Can you work these out from the model? Positions are in its coordinate system, mm. A direction names the side the tool comes from. Coordinates: 2 decimals unless noted, no trailing zeros. Order: outer loops, then holes, each group sorted by start corner. A loop starts at its lowest first (then second) coordinate and runs counter-clockwise, first axis right, second up. Notation, with made-up numbers: (39.25, 14.25) - (83.25, 14.25) arc R17 ccw to (83.25, 39.25) - close; hole circle Ø8 at (14, 51). An arc over 180 degrees is marked (long way). Return JSON: item names as keys, results as strings. Group by question number.
1) Imagine slicing it at A-A (y = 27.02). Write out the boundary of the cut face in (x, z), and give its area (3 significant figures).
2) If I drill on line 1 along Z through (x, y) = (104, 42); line 2 along Y through (x, z) = (33.5, 172.5); line 3 along Z through (x, y) = (64, 43), over which ranges is the centre line in solid material (lowest first)?
3) If we mould it in two halves opening along X, with no side actions, what happens to faces 6 (the face through (9.191, 2.535, 258.964)), 7 (the face through (203.746, 2, 211)), 8 (the face through (154, 2, 266.465))? For each: pulls with the +X half, pulls with the -X half, needs draft (parallel to the pull), parting line crosses it, or undercut.
4) Imagine slicing it at C-C (x = 30). Write out the boundary of the cut face in (y, z), and give its area (3 significant figures).
5) For pin 1 Ø5.5 at (y, z) = (3.5, 272.5) entering from -X; pin 2 Ø1 at (y, z) = (11, 246.5) entering from -X; pin 3 Ø8 at (x, z) = (20, 251.5) entering from -Y; pin 4 Ø8 at (x, z) = (173.5, 82.5) entering from +Y, each with a flat end and sliding along its axis, tell me the tip position at first contact or that it passes through.
6) Which directions (+Z, -Z, +X, -X, +Y, -Y) give clear straight access to the entire face, cutting with the end or side of a thin tool? Please do faces 1 (the face through (17.947, 2.535, 261.535)), 2 (the face through (16, 2.5, 81)), 3 (the face through (88, 49.05, 252)), 4 (the face through (172, 2.5, 81)), 5 (the face through (206, 2, 226.465)).
7) Imagine slicing it at D-D (z = 115). Write out the boundary of the cut face in (x, y), and give its area (4 significant figures).
```python
from build123d import *

# Parameters (mm, degrees)
SKETCH_1_W           = 5
SKETCH_1_H           = 60
SKETCH_1_W_2         = 30
SKETCH_1_H_2         = 5
SKETCH_1_W_3         = 15
EXTRUDE_1_DEPTH      = 5
FILLET_1_R           = 5
SKETCH_2_W           = 245
SKETCH_2_H           = 125
CUT_EXTRUDE_1_DEPTH  = 5
SKETCH_3_W           = 74
SKETCH_3_H           = 2.5
SKETCH_3_W_2         = 73
CUT_EXTRUDE_2_DEPTH  = 10
SKETCH_4_W           = 5
SKETCH_4_H           = 5
CUT_EXTRUDE_3_DEPTH  = 5
SKETCH_5_W           = 50
SKETCH_5_H           = 46.65
EXTRUDE_2_DEPTH      = 47
SKETCH_6_W           = 41.4
SKETCH_6_H           = 44.05
CUT_EXTRUDE_4_DEPTH  = 47
SKETCH_7_R           = 11.25
CUT_EXTRUDE_5_DEPTH  = 317.004529962
CUT_EXTRUDE_6_DEPTH  = 46.65
SKETCH_10_R          = 1.7
CUT_EXTRUDE_7_DEPTH  = 317.004529962
SKETCH_13_R          = 25
CUT_EXTRUDE_9_DEPTH  = 20
FILLET_11_R          = 1.497
CUT_EXTRUDE_10_DEPTH = 358.50996514
SKETCH_17_R          = 2.5
EXTRUDE_3_DEPTH      = 5


with BuildPart() as part:
    # 草圖1 → 填料-伸長1 (new body)
    with BuildSketch(Plane(origin=(0, 0, 0), x_dir=(1, 0, 0), z_dir=(0, 1, 0))):
        Polygon((198.746286718, -286.464902661), (198.746286718, -256.464902661), (183.246286718, -256.464902661), (183.246286718, -266.464902661), (124.746286718, -266.464902661), (124.746286718, -262.464902661), (109.246286718, -262.464902661), (109.246286718, -266.464902661), (-21.253713282, -266.464902661), (-21.253713282, 38.535097339), (-36.253713282, 38.535097339), (-36.253713282, 43.535097339), (203.746286718, 43.535097339), (203.746286718, -286.464902661), align=None)
        with Locations((206.246286718, -256.464902661)):
            Rectangle(SKETCH_1_W, SKETCH_1_H)
        with Locations((206.246286718, 13.535097339)):
            Rectangle(SKETCH_1_W, SKETCH_1_H)
        with Locations((188.746286718, 46.035097339)):
            Rectangle(SKETCH_1_W_2, SKETCH_1_H_2)
        with Locations((-21.253713282, 46.035097339)):
            Rectangle(SKETCH_1_W_2, SKETCH_1_H_2)
        with Locations((91.246286718, 46.035097339)):
            Rectangle(SKETCH_1_W_3, SKETCH_1_H_2)
        with Locations((76.246286718, 46.035097339)):
            Rectangle(SKETCH_1_W_3, SKETCH_1_H_2)
        with Locations((206.246286718, -166.464902661)):
            Rectangle(SKETCH_1_W, SKETCH_1_H)
        with Locations((206.246286718, -76.464902661)):
            Rectangle(SKETCH_1_W, SKETCH_1_H)
    extrude(amount=EXTRUDE_1_DEPTH)

    # 圓角1
    fillet_1_edges = [part.edges().sort_by_distance(p)[0] for p in [
        (208.746286718, 5, -13.535097339),
        (208.746286718, 5, 76.464902661),
        (208.746286718, 5, 166.464902661),
        (208.746286718, 5, 256.464902661),
    ]]
    fillet(fillet_1_edges, radius=FILLET_1_R - 0.0001)  # a hair under: the kernel refuses the full size

    # 草圖2 → 除料-伸長1 (cut)
    with BuildSketch(Plane(origin=(0, 5, 0), x_dir=(1, 0, 0), z_dir=(0, 1, 0))):
        with Locations((86.246286718, -13.964902661)):
            Rectangle(SKETCH_2_W, SKETCH_2_H)
    extrude(amount=-CUT_EXTRUDE_1_DEPTH, mode=Mode.SUBTRACT)

    # 草圖3 → 除料-伸長2 (cut)
    with BuildSketch(Plane(origin=(0, 0, 76.464902661), x_dir=(-1, 0, 0), z_dir=(0, 0, -1))):
        with Locations((-93.746286718, 1.25)):
            Rectangle(SKETCH_3_W, SKETCH_3_H)
        with Locations((-172.246286718, 3.75)):
            Rectangle(SKETCH_3_W_2, SKETCH_3_H)
        with Locations((-15.246286718, 3.75)):
            Rectangle(SKETCH_3_W_2, SKETCH_3_H)
    extrude(amount=-CUT_EXTRUDE_2_DEPTH, mode=Mode.SUBTRACT)

    # 草圖4 → 除料-伸長3 (cut)
    with BuildSketch(Plane(origin=(0, 0, 76.464902661), x_dir=(-1, 0, 0), z_dir=(0, 0, -1))):
        with Locations((-133.246286718, 2.5)):
            Rectangle(SKETCH_4_W, SKETCH_4_H)
        with Locations((-54.246286718, 2.5)):
            Rectangle(SKETCH_4_W, SKETCH_4_H)
    extrude(amount=-CUT_EXTRUDE_3_DEPTH, mode=Mode.SUBTRACT)

    # 草圖5 → 填料-伸長2 (add)
    with BuildSketch(Plane.XY.offset(266.464902661)):
        with Locations((79.746286718, 28.325)):
            Rectangle(SKETCH_5_W, SKETCH_5_H)
    extrude(amount=-EXTRUDE_2_DEPTH)

    # 草圖6 → 除料-伸長4 (cut)
    with BuildSketch(Plane.ZY.offset(-54.746286718)):
        with Locations((242.964902661, 27.025)):
            Rectangle(SKETCH_6_W, SKETCH_6_H)
    extrude(amount=-CUT_EXTRUDE_4_DEPTH, mode=Mode.SUBTRACT)

    # 草圖7 → 除料-伸長5 (cut, through all)
    with BuildSketch(Plane.ZY.offset(-101.746286718)):
        with Locations((242.664902661, 27.02)):
            Circle(SKETCH_7_R)
    extrude(amount=-CUT_EXTRUDE_5_DEPTH, mode=Mode.SUBTRACT)

    # 草圖8 → 除料-伸長6 (cut)
    with BuildSketch(Plane(origin=(0, 51.65, 0), x_dir=(1, 0, 0), z_dir=(0, 1, 0))):
        Polygon((54.746286718, -263.664902661), (101.746286718, -222.464902661), (104.746286718, -222.464902661), (104.746286718, -219.464902661), (54.746286718, -219.464902661), align=None)
    extrude(amount=-CUT_EXTRUDE_6_DEPTH, mode=Mode.SUBTRACT)

    # 草圖10 → 除料-伸長7 (cut, through all)
    with BuildSketch(Plane.ZY.offset(-101.746286718)):
        with Locations((227.164902661, 42.52)):
            Circle(SKETCH_10_R)
        with Locations((258.164902661, 42.52)):
            Circle(SKETCH_10_R)
        with Locations((258.164902661, 11.52)):
            Circle(SKETCH_10_R)
        with Locations((227.164902661, 11.52)):
            Circle(SKETCH_10_R)
    extrude(amount=-CUT_EXTRUDE_7_DEPTH, mode=Mode.SUBTRACT)

    # 草圖13 → 除料-伸長9 (cut)
    with BuildSketch(Plane(origin=(104.746286718, 0, 0), x_dir=(0, 0, -1), z_dir=(1, 0, 0))):
        with Locations((-242.664902661, 27.02)):
            Circle(SKETCH_13_R)
    extrude(amount=CUT_EXTRUDE_9_DEPTH, mode=Mode.SUBTRACT)

    # 圓角11
    fillet_11_edges = [part.edges().sort_by_distance(p)[0] for p in [
        (54.746286718, 28.325, 266.464902661),
        (79.746286718, 51.65, 266.464902661),
        (104.746286718, 28.325, 266.464902661),
        (104.746286718, 27.02, 231.414902661),
        (54.746286718, 51.65, 265.064902661),
        (104.746286718, 51.65, 244.464902661),
        (104.746286718, 28.325, 222.464902661),
        (78.246286718, 51.65, 243.064902661),
        (103.246286718, 51.65, 222.464902661),
    ]]
    fillet(fillet_11_edges, radius=FILLET_11_R)

    # 草圖14 → 除料-伸長10 (cut, through all)
    with BuildSketch(Plane(origin=(0, 5, 0), x_dir=(1, 0, 0), z_dir=(0, 1, 0))):
        Polygon((20.793292101, -266.464902661), (15.019789409, -256.464902661), (3.472784026, -256.464902661), (-2.300718666, -266.464902661), (3.472784026, -276.464902661), (15.019789409, -276.464902661), align=None)
    extrude(amount=-CUT_EXTRUDE_10_DEPTH, mode=Mode.SUBTRACT)

    # 草圖17 → 填料-伸長3 (add)
    with BuildSketch(Plane(origin=(0, 5, 0), x_dir=(1, 0, 0), z_dir=(0, 1, 0))):
        with Locations((9.246286718, -256.464902661)):
            Circle(SKETCH_17_R)
    extrude(amount=-EXTRUDE_3_DEPTH)


solid = part.part
```
Calculated:
{
 "1": {"outline": "(54.75, 263.66) - (101.75, 263.66) - (101.75, 253.91) - (103.25, 253.91) arc R1.5 ccw to (104.75, 255.41) - (104.75, 264.97) arc R1.5 ccw to (103.25, 266.46) - (56.24, 266.46) arc R1.5 ccw to (54.75, 264.97) - close; (101.75, 222.46) - (103.25, 222.46) arc R1.5 ccw to (104.75, 223.96) - (104.75, 229.92) arc R1.5 ccw to (103.25, 231.41) - (101.75, 231.41) - close", "area": "194 mm2"},
 "2": {"line 1": "222.67 to 225.55, 228.78 to 256.55, 259.78 to 266.26", "line 2": "0 to 5", "line 3": "263.66 to 266.46"},
 "3": {"face 6": "undercut", "face 7": "pulls with the +X half", "face 8": "needs draft"},
 "4": {"outline": "(0, 76.46) - (2.5, 76.46) - (2.5, 86.46) - (5, 86.46) - (5, 266.46) - (0, 266.46) - close", "area": "925 mm2"},
 "5": {"pin 1": "x = 198.75", "pin 2": "x = 101.75", "pin 3": "y = 0", "pin 4": "y = 5"},
 "6": {"face 1": "+Z, +Y, -Y", "face 2": "-Z, -X, +Y", "face 3": "-Z, -X", "face 4": "-Z, +X, +Y", "face 5": "+X, +Y, -Y"},
 "7": {"outline": "(-21.25, 0) - (203.75, 0) - (203.75, 5) - (-21.25, 5) - close", "area": "1,125 mm2"}
}
